Design review of the part built by this model. Coordinates are the model's own, in mm. A direction names the side the tool comes from. Round coordinates to 2 decimals unless told otherwise and drop trailing zeros. Order: outer loops, then holes, each group sorted by start corner. A loop starts at its lowest first (then second) coordinate and runs counter-clockwise, first axis right, second up. Notation, with made-up numbers: (15, 56.5) - (28, 56.5) arc R36 ccw to (28, 93.5) - close; hole circle Ø10 at (-27, 77.5). An arc over 180 degrees is marked (long way). Answer as a JSON object with one key per item and string values. Group by question number.
from build123d import *

# Parameters (mm, degrees)
SK_FRONT_W       = 145
SK_FRONT_H       = 140
SK_FRONT_R       = 6
FRONT_DEPTH      = 3
SK_BACK_W        = 127
SK_BACK_H        = 140
BACK_DEPTH       = 3
SK_TOP_W         = 125
SK_TOP_H         = 140
TOP_DEPTH        = 3
SIDE_L_DEPTH     = 3
SIDE_R_DEPTH     = 3
SK_HORN_PLATE_W  = 60
SK_HORN_PLATE_H  = 142
SK_HORN_PLATE_R  = 2
HORN_PLATE_DEPTH = 4


with BuildPart() as part:
    # SK_Front → Front (new body)
    with BuildSketch(Plane(origin=(67, 0, 0), x_dir=(0, 0, -1), z_dir=(1, 0, 0))):
        with Locations((-57.5, 0)):
            Rectangle(SK_FRONT_W, SK_FRONT_H)
        with Locations((-42, 30)):
            Circle(SK_FRONT_R, mode=Mode.SUBTRACT)
        with Locations((-42, -30)):
            Circle(SK_FRONT_R, mode=Mode.SUBTRACT)
    extrude(amount=FRONT_DEPTH)



with BuildPart() as body_2:
    # SK_Back → Back (new body)
    with BuildSketch(Plane(origin=(-55, 0, 0), x_dir=(0, 0, -1), z_dir=(1, 0, 0))):
        with Locations((-66.5, 0)):
            Rectangle(SK_BACK_W, SK_BACK_H)
    extrude(amount=BACK_DEPTH)


with BuildPart() as part_1:
    add(part.part)

    add(body_2.part)  # Top merges body 2
    # SK_Top → Top (add)
    with BuildSketch(Plane.XY.offset(127)):
        with Locations((7.5, 0)):
            Rectangle(SK_TOP_W, SK_TOP_H)
    extrude(amount=TOP_DEPTH)

    # SK_Side_L → Side_L (add)
    with BuildSketch(Plane(origin=(0, 67, 0), x_dir=(1, 0, 0), z_dir=(0, 1, 0))):
        Polygon((-25, 15), (70, 15), (70, -130), (-55, -130), (-55, -3), align=None)
    extrude(amount=SIDE_L_DEPTH)

    # SK_Side_R → Side_R (add)
    with BuildSketch(Plane(origin=(0, -70, 0), x_dir=(1, 0, 0), z_dir=(0, 1, 0))):
        Polygon((-25, 15), (70, 15), (70, -130), (-55, -130), (-55, -3), align=None)
    extrude(amount=SIDE_R_DEPTH)

    # SK_Horn_Plate → Horn_Plate (add)
    with BuildSketch(Plane(origin=(0, 20.5, 0), x_dir=(1, 0, 0), z_dir=(0, 1, 0))):
        with Locations((10, -59)):
            Rectangle(SK_HORN_PLATE_W, SK_HORN_PLATE_H)
        with Locations(Location((0, 0, 0), (0, 0, 270))):
            Circle(SK_HORN_PLATE_R, mode=Mode.SUBTRACT)
    extrude(amount=HORN_PLATE_DEPTH)


solid = part_1.part
1. To check wall thickness, follow line 1 (Y direction, x = -15, z = 21); line 2 (X direction, y = 21, z = 0); line 3 (Y direction, x = 68, z = 42). State the ranges of each line that lie inside material, in increasing order. Write a range as from..to.
2. Take a section at C-C, the plane y = 30. Give the boundary of the cut face in (x, z), then the cut area to 3 significant figures.
3. Take a section at D-D, the plane x = 17. Give the boundary of the cut face in (y, z).
4. Mouldability with a two-part tool opening along Y and no side actions: class faces 1 (the flat face through (40, 22, 58)), 2 (the flat face through (8, 70, 56)), 3 (the flat face through (-40, 68, -6)) as pulls with the +Y half, pulls with the -Y half, needs draft (parallel to the pull), parting line crosses it, or undercut.
5. Tool access review of faces 4 (the flat face through (67, 1, 57)), 5 (the cylindrical face through (-2, 22, 0)), 6 (the flat face through (-40, -69, -6)), 7 (the flat face through (10, 22, -12)), 8 (the cylindrical face through (68.479, 24.143, 43.301)): name each direction out of +Z, -Z, +X, -X, +Y, -Y from which nothing blocks a thin tool from reaching the whole face with its end or side.
6. Take a section at B-B, the plane z = 42. Give the boundary of the cut face in (x, y).
7. Clearance check with flat-ended pins moving along their axes: P1, Ø2.5, axis at x = -53, y = 12, coming from the -Z side; P2, Ø2, axis at x = -3, y = 23, coming from the -Z side; P3, Ø7, axis at y = 30, z = 42, coming from the +X side. State where each tip first meets the part, or that it passes through.
8. Take a section at A-A, the plane z = 8.5. Give the boundary of the cut face in (x, y).
Response values:
{
 "1": {"line 1": "-70..-67, 20.5..24.5, 67..70", "line 2": "-20..-2, 2..40, 67..70", "line 3": "-70..-36, -24..24, 36..70"},
 "2": {"outline": "(-55, 3) - (-52, 3) - (-52, 127) - (67, 127) - (67, 48) - (70, 48) - (70, 130) - (-55, 130) - close; (67, -15) - (70, -15) - (70, 36) - (67, 36) - close", "area": "1,140 mm2"},
 "3": {"outline": "(-70, -15) - (-67, -15) - (-67, 127) - (20.5, 127) - (20.5, -12) - (24.5, -12) - (24.5, 127) - (67, 127) - (67, -15) - (70, -15) - (70, 130) - (-70, 130) - close"},
 "4": {"face 1": "undercut", "face 2": "pulls with the +Y half", "face 3": "needs draft"},
 "5": {"face 4": "-Z", "face 5": "none", "face 6": "-Z, -X, +Y, -Y", "face 7": "-Z, -X", "face 8": "+X"},
 "6": {"outline": "(-55, -70) - (70, -70) - (70, -36) - (67, -36) - (67, -67) - (-52, -67) - (-52, 67) - (67, 67) - (67, 36) - (70, 36) - (70, 70) - (-55, 70) - close; (-20, 20.5) - (40, 20.5) - (40, 24.5) - (-20, 24.5) - close; (67, -24) - (70, -24) - (70, 24) - (67, 24) - close"},
 "7": {"P1": "z = 3", "P2": "z = -12", "P3": "x = -52"},
 "8": {"outline": "(-55, -70) - (70, -70) - (70, 70) - (-55, 70) - close; (-20, 20.5) - (40, 20.5) - (40, 24.5) - (-20, 24.5) - close; hole (-52, -67) - (67, -67) - (67, 67) - (-52, 67) - close"}
}
